from build123d import *

# Parameters (mm, degrees)
SKETCH022_R     = 1
PAD022_DEPTH    = 2.9
SKETCH026_R     = 0.7
SKETCH026_R_2   = 0.5
SKETCH026_W     = 1.3
SKETCH026_H     = 0.5
POCKET009_DEPTH = 0.6
SKETCH027_R     = 0.7
SKETCH027_W     = 1.3
SKETCH027_H     = 0.5
POCKET010_DEPTH = 0.6


with BuildPart() as part:
    # Sketch022 → Pad022 (new body, symmetric)
    with BuildSketch(Plane.XZ):
        Polygon((-6.4, -1.15), (-4.3, -1.15), (-3.95, -1.5), (-1.95, -1.5), (-1.6, -1.15), (1.6, -1.15), (1.95, -1.5), (3.95, -1.5), (4.3, -1.15), (6.4, -1.15), (6.4, 1.35), (5.8, 1.35), (5.8, 2.2), (4.65, 2.2), (4.65, 1.7), (1.6, 1.7), (1.25, 1.35), (-1.25, 1.35), (-1.6, 1.7), (-5.8, 1.7), (-5.8, 1.35), (-6.4, 1.35), align=None)
        with Locations((-3.25, 0)):
            Circle(SKETCH022_R, mode=Mode.SUBTRACT)
        with Locations((3.25, 0)):
            Circle(SKETCH022_R, mode=Mode.SUBTRACT)
    extrude(amount=PAD022_DEPTH, both=True)

    # Sketch026 (on Face26 of Pad022) → Pocket009 (cut)
    with BuildSketch(Plane.XZ.offset(2.9)):
        with Locations((-5.3, 0)):
            Circle(SKETCH026_R)
        with Locations((5.1, 0)):
            Circle(SKETCH026_R_2)
        Polygon((1.75, 1.35), (1.75, -0.75), (-1.75, -0.75), (-1.75, 1.35), (-6.4, 1.35), (-6.4, 2.2), (6.4, 2.2), (6.4, 1.35), align=None)
        with Locations((0, 0.4)):
            Rectangle(SKETCH026_W, SKETCH026_H, mode=Mode.SUBTRACT)
    extrude(amount=-POCKET009_DEPTH, mode=Mode.SUBTRACT)

    # Sketch027 (on Face4 of Pocket009) → Pocket010 (cut)
    with BuildSketch(Plane(origin=(0, 2.9, 0), x_dir=(1, 0, 0), z_dir=(0, 1, 0))):
        with Locations((5.3, 0)):
            Circle(SKETCH027_R)
        with Locations((-5.3, 0)):
            Circle(SKETCH027_R)
        Polygon((1.75, 0.75), (-1.75, 0.75), (-1.75, -1.35), (-6.4, -1.35), (-6.4, -2.2), (6.4, -2.2), (6.4, -1.35), (1.75, -1.35), align=None)
        with Locations((0, -0.4)):
            Rectangle(SKETCH027_W, SKETCH027_H, mode=Mode.SUBTRACT)
    extrude(amount=-POCKET010_DEPTH, mode=Mode.SUBTRACT)


solid = part.part
Check sheet for the modelled part. Datum: model origin and axes. Units: mm. A direction names the side the tool comes from. Round coordinates to 2 decimals unless told otherwise and drop trailing zeros. Loops run counter-clockwise (first coordinate to the right, second up) from the corner with the lowest first, then second, coordinate; pieces in that order, holes last. Notation, with made-up numbers: (18.25, -18) -> (42.25, -18) arc R16 cw to (42.25, 8) -> close; hole circle Ø10 at (26, 69.25). An arc over 180 degrees is marked (long way). Put each result on its own line as item: value. Start each with the question number.
1. Section check B-B (y = 0.5). Enter the section's corners in (x, z), plus the area to 3 significant figures.
2. Section check D-D (x = -5.3). Enter the section's corners in (y, z).
3. Section check C-C (z = 1.5). Enter the section's corners in (x, y).
4. Access from +Z, -Z, +X, -X, +Y, -Y to the whole of each face (thin tool, end or side, straight path). Record for faces 1 (the face through (6, 0, 1.35)), 2 (the face through (3, 0, 1.7)), 3 (the face through (5, -2.3, 0)), 4 (the face through (5.8, 0, 2)).
5. Section check A-A (x = -3.25). Enter the section's corners in (y, z).
6. Scan lines: probe 1 along Z at (x, y) = (-3.25, 1.3); probe 2 along Z at (x, y) = (5.3, 2.65); probe 3 along Z at (x, y) = (-4.5, 2.35). Record each from-to range of solid material in increasing order.
7. Draft check along X on faces 5 (the face through (6.4, 0, 0)), 6 (the face through (-2, -2.9, -1)), 7 (the face through (-6, -2.6, 0)). Enter one of: +X half, -X half, draft (parallel to the pull), parting line (faces both ways), or undercut.
8. Gauge pin test, flat ends, axial feed: pin 1 (1 mm diameter, centred on x = -0.5, y = 0, fed in from -Z); pin 2 (2.5 mm diameter, centred on x = -4.5, y = 1, fed in from +Z). Record the tip position at first contact, or that the pin passes through.
Findings:
1. outline: (-6.4, -1.15) -> (-4.3, -1.15) -> (-3.95, -1.5) -> (-1.95, -1.5) -> (-1.6, -1.15) -> (1.6, -1.15) -> (1.95, -1.5) -> (3.95, -1.5) -> (4.3, -1.15) -> (6.4, -1.15) -> (6.4, 1.35) -> (5.8, 1.35) -> (5.8, 2.2) -> (4.65, 2.2) -> (4.65, 1.7) -> (1.6, 1.7) -> (1.25, 1.35) -> (-1.25, 1.35) -> (-1.6, 1.7) -> (-5.8, 1.7) -> (-5.8, 1.35) -> (-6.4, 1.35) -> close; hole circle Ø2 at (-3.25, 0); hole circle Ø2 at (3.25, 0)
1. area: 31.0 mm^2
2. outline: (-2.9, -1.15) -> (2.9, -1.15) -> (2.9, -0.7) -> (2.3, -0.7) -> (2.3, 0.7) -> (2.9, 0.7) -> (2.9, 1.35) -> (2.3, 1.35) -> (2.3, 1.7) -> (-2.3, 1.7) -> (-2.3, 1.35) -> (-2.9, 1.35) -> (-2.9, 0.7) -> (-2.3, 0.7) -> (-2.3, -0.7) -> (-2.9, -0.7) -> close
3. outline: (-5.8, -2.3) -> (-1.4, -2.3) -> (-1.4, 2.3) -> (-5.8, 2.3) -> close; (1.4, -2.3) -> (5.8, -2.3) -> (5.8, 2.3) -> (1.4, 2.3) -> close
4. face 1: +Z, +X
4. face 2: +Z, -X, +Y, -Y
4. face 3: -Y
4. face 4: +Z, +X, +Y, -Y
5. outline: (-2.9, -1.5) -> (2.9, -1.5) -> (2.9, -1) -> (-2.9, -1) -> close; (-2.9, 1) -> (2.9, 1) -> (2.9, 1.35) -> (2.3, 1.35) -> (2.3, 1.7) -> (-2.3, 1.7) -> (-2.3, 1.35) -> (-2.9, 1.35) -> close
6. probe 1: z = -1.5 to -1, 1 to 1.7
6. probe 2: z = -1.15 to -0.7, 0.7 to 1.35
6. probe 3: z = -1.15 to 1.35
7. face 5: +X half
7. face 6: draft
7. face 7: undercut
8. pin 1: stops at z = -1.15
8. pin 2: stops at z = 1.7
